Verification items for the finished model (mm, model axes). A direction names the side the tool comes from. Give positions to 0.01 mm unless a question says otherwise; leave off trailing zeros. Order: outer loops, then holes, each group sorted by start corner. A loop starts at its lowest first (then second) coordinate and runs counter-clockwise, first axis right, second up.
(1) Access from +Z, -Z, +X, -X, +Y, -Y to the whole of each face (thin tool, end or side, straight path). Record for faces 4 (the face through (5.158, -3.955, 16.779)), 5 (the face through (-8, 0, 13.3)), 6 (the face through (0, -4.8, -3)), 7 (the face through (7.45, 0, 7)).
(2) Sectioned sample at C-C on x = 0. Record the cut outline in (y, z), plus the area to 3 significant figures.
(3) Gauge pin test, flat ends, axial feed: pin 1 (4 mm diameter, centred on y = -2, z = 2, fed in from +X); pin 2 (4.5 mm diameter, centred on x = 2.5, y = -2.5, fed in from +Z); pin 3 (0.5 mm diameter, centred on y = 4.5, z = -3.5, fed in from +X); pin 4 (1 mm diameter, centred on x = 3, y = -4, fed in from +Z). Record the tip position at first contact, or that the pin passes through.
(4) Scan lines: L1, parallel to X at y = -4.5, z = -4.5; L2, parallel to Z at x = 0.5, y = 7; L3, parallel to Y at x = 0.25, z = 17. Record each from-to range of solid material in increasing order.
(5) Mould release check, pull along Y, two halves, no side actions. Record for faces 1 (the face through (0, 4.2, -3)), 2 (the face through (0.39, -1.77, 18.77)), 3 (the face through (0, 4.8, -3)): pulls with the +Y half, pulls with the -Y half, needs draft (parallel to the pull), parting line crosses it, or undercut.
(6) Sectioned sample at B-B on y = 0. Record the cut outline in (x, z), plus the area to 3 significant figures.
(7) Sectioned sample at A-A on z = -1. Record the cut outline in (x, y).
Autodesk Fusion 360 part; units mm, degrees
sketch "Sketch1" plane through (0, 0, 0) normal (0, 0, 1) x (1, 0, 0)
  circle A0 centre (0, 0) radius 8
  line L0 (7.45, -9) -> (-7.45, -9)
  line L1 (-7.45, -9) -> (-7.45, 9)
  line L2 (-7.45, 9) -> (7.45, 9)
  line L3 (7.45, 9) -> (7.45, -9)
  line L4 (7.45, -9) -> (-7.45, 9) construction
  line L5 (-7.45, -9) -> (7.45, 9) construction
  dimension "d1" = 16
  dimension "d2" = 14.9
extrude "Extrude1" add sketch "Sketch1" along normal blind 13.3 contours A0 L1 L3
sketch "Sketch2" plane through (0, 0, 13.3) normal (0, 0, 1) x (-1, 0, 0)
  arc A0 (7.45, 2.915) -> (-7.45, 2.915) centre (0, 0) ccw
  line L0 (-7.45, 2.915) -> (-7.45, -2.915)
  arc A1 (-7.45, -2.915) -> (7.45, -2.915) centre (0, 0) ccw
  line L1 (7.45, -2.915) -> (7.45, 2.915)
  circle A2 centre (0, 0) radius 9.45
  dimension "d5" = 18.9
extrude "Extrude2" add sketch "Sketch2" along normal blind 2 contours A0 L0 A1 L1 | A2
chamfer "Chamfer1" distance 2 distance2 1 1 edges at (8.8105, 3.4173, 15.3) measured on face at (-3.5181, 1.5655, 15.3)
sketch "Sketch3" plane through (0, 0, 15.3) normal (0, 0, 1) x (-1, 0, 0)
  circle A0 centre (0, 0) radius 7.45
  circle A1 centre (0, 0) radius 6.5
  dimension "d10" = 13
extrude "Extrude3" add sketch "Sketch3" along normal blind 3.5 contours A1
chamfer "Chamfer2" distance 5 distance2 0.5 1 edges at (6.0601, 2.3505, 18.8) measured on face at (-1.9521, 0.9401, 18.8)
sketch "Sketch4" plane through (0, 0, 0) normal (0, 0, -1) x (1, 0, 0)
  arc A0 (7.45, 2.915) -> (-7.45, 2.915) centre (0, 0) ccw
  line L0 (-7.45, 2.915) -> (-7.45, -2.915)
  arc A1 (-7.45, -2.915) -> (7.45, -2.915) centre (0, 0) ccw
  line L1 (7.45, -2.915) -> (7.45, 2.915)
  line L2 (0, 8) -> (0, 4.8) construction
  line L3 (0, -8) -> (0, -4.8) construction
  line L4 (0, -4.8) -> (0, -4.2) construction
  line L5 (0, 4.8) -> (0, 4.2) construction
  line L6 (1.45, 4.2) -> (-1.45, 4.2)
  line L7 (-1.45, 4.2) -> (-1.45, 4.8)
  line L8 (-1.45, 4.8) -> (1.45, 4.8)
  line L9 (1.45, 4.8) -> (1.45, 4.2)
  line L10 (1.45, 4.2) -> (-1.45, 4.8) construction
  line L11 (-1.45, 4.2) -> (1.45, 4.8) construction
  line L12 (1.45, -4.8) -> (-1.45, -4.8)
  line L13 (-1.45, -4.8) -> (-1.45, -4.2)
  line L14 (-1.45, -4.2) -> (1.45, -4.2)
  line L15 (1.45, -4.2) -> (1.45, -4.8)
  line L16 (1.45, -4.8) -> (-1.45, -4.2) construction
  line L17 (-1.45, -4.8) -> (1.45, -4.2) construction
  point P0 (0, 4.5)
  point P1 (0, -4.5)
  dimension "d15" = 3.2
  dimension "d16" = 3.2
  dimension "d17" = 0.6
  dimension "d18" = 0.6
  dimension "d19" = 2.9
  dimension "d20" = 0.6
  dimension "d21" = 2.9
  dimension "d22" = 0.6
extrude "Extrude4" add sketch "Sketch4" along normal blind 5.7 contours L6 L7 L8 L9 | L12 L13 L14 L15
Ans:
1. face 4: +Z
1. face 5: -Z
1. face 6: -Z, +X, -X, -Y
1. face 7: -Z, +X, +Y, -Y
2. outline: (-9.45, 13.3) - (-8, 13.3) - (-8, 0) - (-4.8, 0) - (-4.8, -5.7) - (-4.2, -5.7) - (-4.2, 0) - (4.2, 0) - (4.2, -5.7) - (4.8, -5.7) - (4.8, 0) - (8, 0) - (8, 13.3) - (9.45, 13.3) - (9.45, 14.3) - (7.45, 15.3) - (6.5, 15.3) - (6.5, 18.3) - (1.5, 18.8) - (-1.5, 18.8) - (-6.5, 18.3) - (-6.5, 15.3) - (-7.45, 15.3) - (-9.45, 14.3) - close
2. area: 298 mm2
3. pin 1: stops at x = 7.45
3. pin 2: stops at z = 18.8
3. pin 3: stops at x = 1.45
3. pin 4: stops at z = 18.5
4. L1: x = -1.45 to 1.45
4. L2: z = 0 to 15.3
4. L3: y = -6.5 to 6.5
5. face 1: undercut
5. face 2: parting line crosses it
5. face 3: pulls with the +Y half
6. outline: (-9.45, 13.3) - (-7.45, 13.3) - (-7.45, 0) - (7.45, 0) - (7.45, 13.3) - (9.45, 13.3) - (9.45, 14.3) - (7.45, 15.3) - (6.5, 15.3) - (6.5, 18.3) - (1.5, 18.8) - (-1.5, 18.8) - (-6.5, 18.3) - (-6.5, 15.3) - (-7.45, 15.3) - (-9.45, 14.3) - close
6. area: 277 mm2
7. outline: (-1.45, -4.8) - (1.45, -4.8) - (1.45, -4.2) - (-1.45, -4.2) - close; (-1.45, 4.2) - (1.45, 4.2) - (1.45, 4.8) - (-1.45, 4.8) - close
